Build history of the part. All positions in model axes, mm. A direction names the side the tool comes from. Round coordinates to 2 decimals unless told otherwise and drop trailing zeros. Write each loop counter-clockwise with the first axis right and the second up, starting at its lowest first coordinate (ties: lowest second). Pieces come first, ordered by that corner, then holes. Notation, with made-up numbers: M -3,23.25 L 25,23.25 A9 cw 25,32.25 Z; hole C 47.5,16.25 d7. An arc over 180 degrees is marked long. Write item = value, one per line.
from build123d import *

# Parameters (mm, degrees)
SKETCH1_R           = 1.5
BOSS_EXTRUDE1_DEPTH = 5


with BuildPart() as part:
    # Sketch1 → Boss-Extrude1 (new body)
    with BuildSketch(Plane(origin=(0, 0, 0), x_dir=(1, 0, 0), z_dir=(0, 1, 0))):
        with BuildLine():
            Line((-57.5, 37.5), (57.5, 37.5))
            ThreePointArc((57.5, 37.5), (95, 0), (57.5, -37.5))
            Line((57.5, -37.5), (30, -37.5))
            Line((30, -37.5), (30, -12.5))
            Line((30, -12.5), (-30, -12.5))
            Line((-30, -12.5), (-30, -37.5))
            Line((-30, -37.5), (-57.5, -37.5))
            ThreePointArc((-57.5, -37.5), (-95, 0), (-57.5, 37.5))
        make_face()
        with Locations(Location((-90, 0, 0), (0, 0, 270))):
            Circle(SKETCH1_R, mode=Mode.SUBTRACT)
        with Locations(Location((-30, 32.5, 0), (0, 0, 270))):
            Circle(SKETCH1_R, mode=Mode.SUBTRACT)
        with Locations(Location((30, 32.5, 0), (0, 0, 270))):
            Circle(SKETCH1_R, mode=Mode.SUBTRACT)
        with Locations(Location((90, 0, 0), (0, 0, 270))):
            Circle(SKETCH1_R, mode=Mode.SUBTRACT)
        with Locations(Location((34.949747468, -30.550252532, 0), (0, 0, 270))):
            Circle(SKETCH1_R, mode=Mode.SUBTRACT)
        with Locations(Location((-34.949747468, -30.550252532, 0), (0, 0, 270))):
            Circle(SKETCH1_R, mode=Mode.SUBTRACT)
    extrude(amount=BOSS_EXTRUDE1_DEPTH)


solid = part.part
1. Tool access for faces 5 (the face through (44, 2, 37.5)), 6 (the face through (-30, 2, 25)): list every direction of +Z, -Z, +X, -X, +Y, -Y with a clear straight run to the whole face (end or side of a thin tool).
Responses:
face_5 = +Z, +X, -X, +Y, -Y
face_6 = +Z, +Y, -Y
2. Band-saw the part on A-A (y = 4). List the corners of the cut face in (x, z).
Responses:
outline = M -57.5,-37.5 L 57.5,-37.5 A37.5 ccw 57.5,37.5 L 30,37.5 L 30,12.5 L -30,12.5 L -30,37.5 L -57.5,37.5 A37.5 ccw Z; hole C -90,0 d3; hole C -34.95,30.55 d3; hole C -30,-32.5 d3; hole C 30,-32.5 d3; hole C 34.95,30.55 d3; hole C 90,0 d3
3. Band-saw the part on B-B (z = -22.5). List the corners of the cut face in (x, y).
Responses:
outline = M -87.5,0 L 87.5,0 L 87.5,5 L -87.5,5 Z
4. Flat gauge pins, fed straight in: pin 1 (2.5 mm diameter, centred on x = -90, z = 0, fed in from +Y); pin 2 (2.5 mm diameter, centred on x = 1.5, y = 3, fed in from +Z); pin 3 (1.5 mm diameter, centred on y = 1.5, z = 22.5, fed in from +X); pin 4 (2.5 mm diameter, centred on y = 2.5, z = 31, fed in from -X). Where does each tip first touch, or does it go through?
Responses:
pin_1 = through
pin_2 = 12.5
pin_3 = 88.05
pin_4 = -80.33
5. Probe probe 1 along X at (y, z) = (2.25, 0); probe 2 along X at (y, z) = (3.8, -32.5); probe 3 along X at (y, z) = (3.8, 15). List the from-to ranges inside material, lowest first.
Responses:
probe_1 = -95 to -91.5, -88.5 to 88.5, 91.5 to 95
probe_2 = -76.21 to -31.5, -28.5 to 28.5, 31.5 to 76.21
probe_3 = -91.87 to -30, 30 to 91.87
6. Band-saw the part on C-C (x = 67.5). List the corners of the cut face in (y, z), plus the area to 3 significant figures.
Responses:
outline = M 0,-36.14 L 5,-36.14 L 5,36.14 L 0,36.14 Z
area = 361 mm²
7. Mould opens along X. For faces 1 (the face through (-1, 2, -37.5)), 2 (the face through (94.99, 2.46, -0.82)), 3 (the face through (0, 2, 12.5)), 4 (the face through (-94.99, 2.46, 0.82)) say: pulls with the +X half, pulls with the -X half, needs draft (parallel to the pull), parting line crosses it, or undercut.
Responses:
face_1 = needs draft
face_2 = pulls with the +X half
face_3 = undercut
face_4 = pulls with the -X half
